CAD build for the part. Positions are in the model's coordinates, mm. Face numbers are marked on the shaded views. A direction names the side the tool comes from. Round coordinates to 2 decimals unless told otherwise and drop trailing zeros. Order: outer loops, then holes, each group sorted by start corner. A loop starts at its lowest first (then second) coordinate and runs counter-clockwise, first axis right, second up.
```python
from build123d import *

# Parameters (mm, degrees)
BOSS_EXTRUDE1_DEPTH = 25.4
SKETCH4_W           = 26
SKETCH4_H           = 25.4
CUT_EXTRUDE3_DEPTH  = 5.08


with BuildPart() as part:
    # Sketch1 → Boss-Extrude1 (new body)
    with BuildSketch(Plane.XY):
        with BuildLine():
            Line((0, 0), (79.31147458, 0))
            ThreePointArc((79.31147458, 0), (39.65573729, -19.05), (0, 0))
        make_face()
    extrude(amount=BOSS_EXTRUDE1_DEPTH)

    # Sketch4 → Cut-Extrude3 (cut)
    with BuildSketch(Plane(origin=(0, 0, 0), x_dir=(1, 0, 0), z_dir=(0, 1, 0))):
        with Locations((39.65573729, -12.7)):
            Rectangle(SKETCH4_W, SKETCH4_H)
    extrude(amount=-CUT_EXTRUDE3_DEPTH, mode=Mode.SUBTRACT)


solid = part.part
```
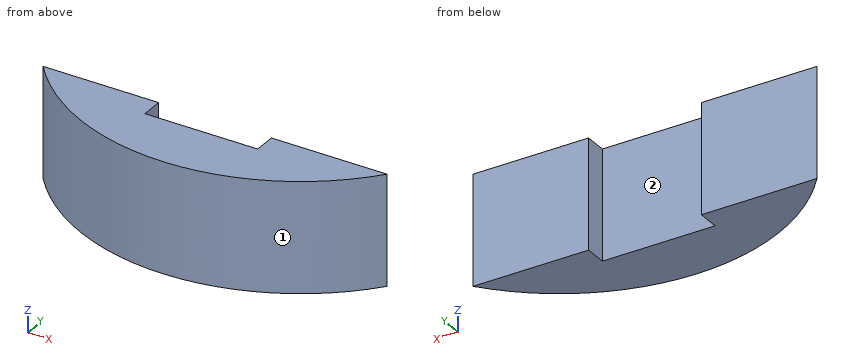
1. Cut at C-C, the plane x = 10.5. Write the cut outline in (y, z).
2. Tool access for the marked faces 1 and 2: list every direction of +Z, -Z, +X, -X, +Y, -Y with a clear straight run to the whole face (end or side of a thin tool).
3. Cut at A-A, the plane y = -3.25. Write the cut outline in (x, z).
4. Drill centre lines: line 1 (X direction, y = -4.25, z = 15.25); line 2 (X direction, y = -1, z = 6.25); line 3 (X direction, y = -10, z = 21.5). Where is each one in solid material? Low to high.
5. Cut at B-B, the plane z = 10. Write the cut outline in (x, y).
6. Pin check, flat tips, straight feed: P1, Ø10, axis at y = -8.5, z = 19, coming from the +X side; P2, Ø2.5, axis at y = -3.5, z = 6.5, coming from the +X side; P3, Ø4, axis at x = 65.5, z = 16, coming from the -Y side. Stop position of each tip, or through.
7. Cut at D-D, the plane y = -17. Write the cut outline in (x, z), and give its area (3 significant figures).
Outcome:
1. outline: (-9.85, 0) - (0, 0) - (0, 25.4) - (-9.85, 25.4) - close
2. face 1: +Z, -Z, -Y
2. face 2: +Z, -Z, +Y
3. outline: (2.84, 0) - (26.66, 0) - (26.66, 25.4) - (2.84, 25.4) - close; (52.66, 0) - (76.47, 0) - (76.47, 25.4) - (52.66, 25.4) - close
4. line 1: x = 3.81 to 26.66, 52.66 to 75.5
4. line 2: x = 0.82 to 26.66, 52.66 to 78.49
4. line 3: x = 10.71 to 68.6
5. outline: (0, 0) arc R50.8 ccw to (79.31, 0) - (52.66, 0) - (52.66, -5.08) - (26.66, -5.08) - (26.66, 0) - close
6. P1: stops at x = 76.24
6. P2: stops at x = 77.4
6. P3: stops at y = -13.11
7. outline: (25.37, 0) - (53.94, 0) - (53.94, 25.4) - (25.37, 25.4) - close
7. area: 726 mm2
